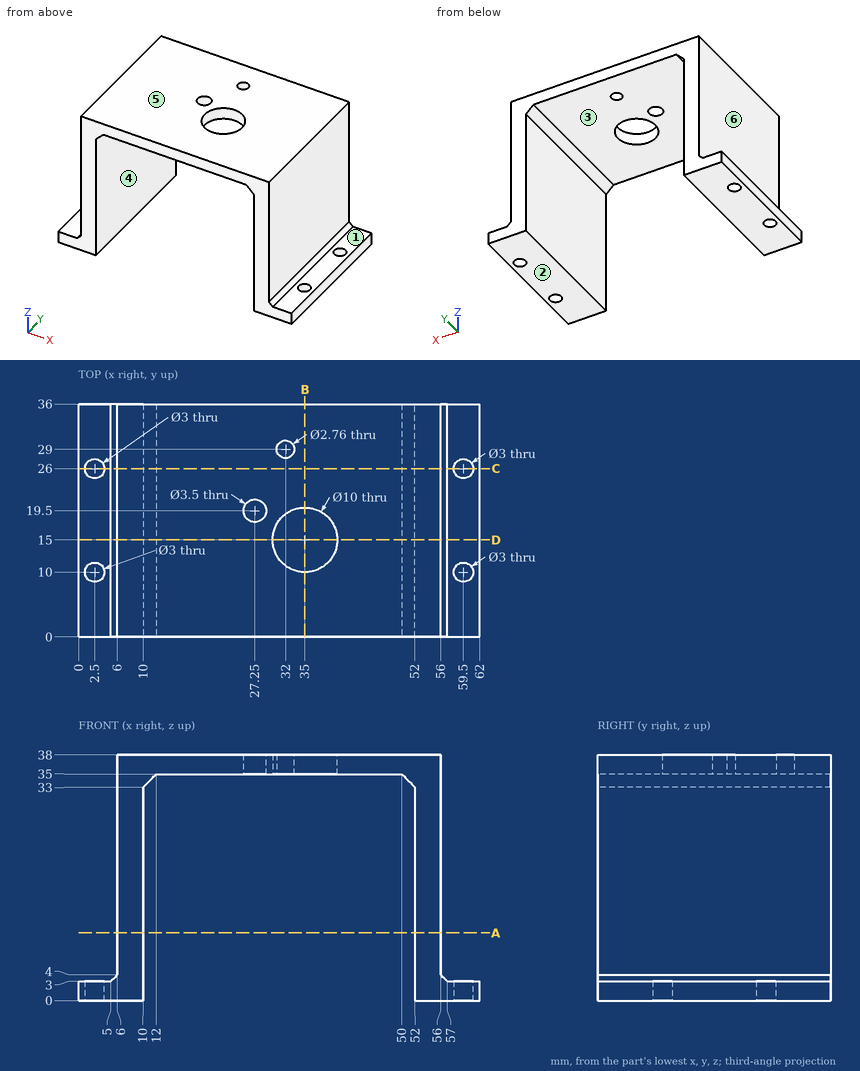
Could you check a few things on this drawing? It's one solid part, dimensions in mm from its lowest x, y, z. A direction names the side the tool comes from. Give positions to 0.01 mm unless a question says otherwise; leave off trailing zeros. Order: outer loops, then holes, each group sorted by start corner. A loop starts at its lowest first (then second) coordinate and runs counter-clockwise, first axis right, second up.
1. Suppose I cut it at C-C (y = 26). Write out the boundary of the cut face in (x, z), plus the area to 3 significant figures.
Answers below:
outline: (0, 0) - (1, 0) - (1, 3) - (0, 3) - close; (4, 0) - (10, 0) - (10, 33) - (12, 35) - (50, 35) - (52, 33) - (52, 0) - (58, 0) - (58, 3) - (57, 3) - (56, 4) - (56, 38) - (6, 38) - (6, 4) - (5, 3) - (4, 3) - close; (61, 0) - (62, 0) - (62, 3) - (61, 3) - close
area: 453 mm2
2. For pin 1 (18 mm diameter, centred on x = 35, y = 25, fed in from -Z); pin 2 (10 mm diameter, centred on y = 26.5, z = 25, fed in from -X); pin 3 (5.5 mm diameter, centred on x = 60.5, y = 19.5, fed in from +Z); pin 4 (2 mm diameter, centred on x = 27.25, y = 19.5, fed in from +Z), each with a flat end and sliding along its axis, tell me the tip position at first contact or that it passes through.
Answers below:
pin 1: stops at z = 35
pin 2: stops at x = 6
pin 3: stops at z = 3
pin 4: passes through
3. Thinking about a two-plate mould opening in X: for the marked faces 4, 5 and 6, which applies, +X half, -X half, draft (parallel to the pull), parting line (faces both ways), or undercut?
Answers below:
face 4: undercut
face 5: draft
face 6: -X half
4. Suppose I cut it at B-B (x = 35). Write out the boundary of the cut face in (y, z), plus the area to 3 significant figures.
Answers below:
outline: (0, 35) - (10, 35) - (10, 38) - (0, 38) - close; (20, 35) - (36, 35) - (36, 38) - (20, 38) - close
area: 78.0 mm2
5. Suppose I cut it at D-D (y = 15). Write out the boundary of the cut face in (x, z).
Answers below:
outline: (0, 0) - (10, 0) - (10, 33) - (12, 35) - (30, 35) - (30, 38) - (6, 38) - (6, 4) - (5, 3) - (0, 3) - close; (40, 35) - (50, 35) - (52, 33) - (52, 0) - (62, 0) - (62, 3) - (57, 3) - (56, 4) - (56, 38) - (40, 38) - close
6. Which directions (+Z, -Z, +X, -X, +Y, -Y) give clear straight access to the entire face, cutting with the end or side of a thin tool? Please do the marked faces 1, 2 and 3.
Answers below:
face 1: +Z, +X, +Y, -Y
face 2: -Z, +X, -X, +Y, -Y
face 3: -Z, +Y, -Y
7. I need wall thicknesses on L1, parallel to X at y = 26, z = 1.85; L2, parallel to X at y = 8, z = 30.5; L3, parallel to Y at x = 2, z = 1. Which ranges of each line are inside material? Lowest first, please.
Answers below:
L1: x = 0 to 1, 4 to 10, 52 to 58, 61 to 62
L2: x = 6 to 10, 52 to 56
L3: y = 0 to 8.59, 11.41 to 24.59, 27.41 to 36
8. Suppose I cut it at A-A (z = 10.5). Write out the boundary of the cut face in (x, y).
Answers below:
outline: (6, 0) - (10, 0) - (10, 36) - (6, 36) - close; (52, 0) - (56, 0) - (56, 36) - (52, 36) - close
